```python
from build123d import *

# Parameters (mm, degrees)
SKETCH_3_R      = 1.6
EXTRUDE_2_DEPTH = 4


with BuildPart() as part:
    # Эскиз3 → Бобышка-Вытянуть2 (new body)
    # profile 1 of 6: a face of its own
    with BuildSketch(Plane.XY):
        Polygon((-16, -10), (-70, -10), (-70, -15.5), (-57.5, -15.5), (-57.5, -36.5), (-70, -36.5), (-70, -42), (-16, -42), (-16, -36.5), (-28.5, -36.5), (-28.5, -15.5), (-16, -15.5), align=None)
        with Locations((-66, -39)):
            Circle(SKETCH_3_R, mode=Mode.SUBTRACT)
        with Locations((-54, -26)):
            Circle(SKETCH_3_R, mode=Mode.SUBTRACT)
        with Locations((-20, -39)):
            Circle(SKETCH_3_R, mode=Mode.SUBTRACT)
        with Locations((-32, -26)):
            Circle(SKETCH_3_R, mode=Mode.SUBTRACT)
        with Locations((-66, -13)):
            Circle(SKETCH_3_R, mode=Mode.SUBTRACT)
        with Locations((-20, -13)):
            Circle(SKETCH_3_R, mode=Mode.SUBTRACT)
    # profile 2 of 6: a face of its own
    with BuildSketch(Plane.XY):
        Polygon((70, -10), (43, -10), (43, -42), (70, -42), (70, -36.5), (57.5, -36.5), (57.5, -15.5), (70, -15.5), align=None)
        with Locations((66, -39)):
            Circle(SKETCH_3_R, mode=Mode.SUBTRACT)
        with Locations((54, -26)):
            Circle(SKETCH_3_R, mode=Mode.SUBTRACT)
        with Locations((66, -13)):
            Circle(SKETCH_3_R, mode=Mode.SUBTRACT)
    # profile 3 of 6: a face of its own
    with BuildSketch(Plane.XY):
        Polygon((-70, 10), (-70, -10), (-16, -10), (43, -10), (70, -10), (70, 10), (43, 10), (-16, 10), (-43, 10), align=None)
    # profile 4 of 6: a face of its own
    with BuildSketch(Plane.XY):
        Polygon((-43, 42), (-43, 10), (-16, 10), (-16, 15.5), (-28.5, 15.5), (-28.5, 36.5), (-16, 36.5), (-16, 42), align=None)
        with Locations((-20, 13)):
            Circle(SKETCH_3_R, mode=Mode.SUBTRACT)
        with Locations((-32, 26)):
            Circle(SKETCH_3_R, mode=Mode.SUBTRACT)
        with Locations((-20, 39)):
            Circle(SKETCH_3_R, mode=Mode.SUBTRACT)
    # profile 5 of 6: a face of its own
    with BuildSketch(Plane.XY):
        Polygon((-70, 15.5), (-70, 10), (-43, 10), (-43, 42), (-70, 42), (-70, 36.5), (-57.5, 36.5), (-57.5, 15.5), align=None)
        with Locations((-66, 13)):
            Circle(SKETCH_3_R, mode=Mode.SUBTRACT)
        with Locations((-54, 26)):
            Circle(SKETCH_3_R, mode=Mode.SUBTRACT)
        with Locations((-66, 39)):
            Circle(SKETCH_3_R, mode=Mode.SUBTRACT)
    # profile 6 of 6: a face of its own
    with BuildSketch(Plane.XY):
        Polygon((43, 10), (70, 10), (70, 15.5), (57.5, 15.5), (57.5, 36.5), (70, 36.5), (70, 42), (43, 42), align=None)
        with Locations((66, 13)):
            Circle(SKETCH_3_R, mode=Mode.SUBTRACT)
        with Locations((54, 26)):
            Circle(SKETCH_3_R, mode=Mode.SUBTRACT)
        with Locations((66, 39)):
            Circle(SKETCH_3_R, mode=Mode.SUBTRACT)
    extrude(amount=EXTRUDE_2_DEPTH)


solid = part.part
```
Model file for the job. Use its own axes, mm. A direction names the side the tool comes from. Coordinates: 2 decimals unless noted, no trailing zeros. Write each loop counter-clockwise with the first axis right and the second up, starting at its lowest first coordinate (ties: lowest second). Pieces come first, ordered by that corner, then holes. Notation, with made-up numbers: (-35.75, 77) - (-19.75, 77) arc R9 cw to (-19.75, 81) - close; hole circle Ø2 at (-7.5, 12). An arc over 180 degrees is marked (long way). One line per item, written item: value. Start each with the question number.
1. Mould opens along Y. For faces 1 (the flat face through (-43, -42, 2)), 2 (the cylindrical face through (-64.52, 38.39, 1.97)), 3 (the flat face through (-16, -39, 2)) say: released by +Y, released by -Y, zero draft, split by the parting line, or undercut.
2. Slice it at A-A (x = 54). Write the cut outline in (y, z).
3. Tool access for faces 4 (the flat face through (-28.5, -26, 2)), 5 (the flat face through (70, 0, 2)), 6 (the flat face through (57, 42, 2)), 7 (the flat face through (43, 26, 2)), 8 (the flat face through (-16, -13, 2)): list every direction of +Z, -Z, +X, -X, +Y, -Y with a clear straight run to the whole face (end or side of a thin tool).
4. Slice it at B-B (y = 26). Write the cut outline in (x, z).
5. Probe line 1 (Y direction, x = -54, z = 1.35); line 2 (X direction, y = -10.5, z = 1.1); line 3 (X direction, y = -12, z = 0.65). List the from-to ranges inside material, lowest first. Write a range as from..to.
6. Flat gauge pin, fed straight in: pin 1 (1.2 mm diameter, centred on x = -0.5, z = 3, fed in from +Y). Where does the tip first touch, or does it go through?
7. Slice it at D-D (z = 3.1). Count the separate pieces of the cut face and the enclosed holes in it, plus the area to 3 significant figures.
8. Slice it at C-C (y = -39). Write the cut outline in (x, z), plus the area to 3 significant figures.
Answers below:
1. face 1: released by -Y
1. face 2: undercut
1. face 3: zero draft
2. outline: (-42, 0) - (-27.6, 0) - (-27.6, 4) - (-42, 4) - close; (-24.4, 0) - (24.4, 0) - (24.4, 4) - (-24.4, 4) - close; (27.6, 0) - (42, 0) - (42, 4) - (27.6, 4) - close
3. face 4: +Z, -Z
3. face 5: +Z, -Z, +X, +Y, -Y
3. face 6: +Z, -Z, +X, -X, +Y
3. face 7: +Z, -Z, +Y
3. face 8: +Z, -Z, -Y
4. outline: (-57.5, 0) - (-55.6, 0) - (-55.6, 4) - (-57.5, 4) - close; (-52.4, 0) - (-33.6, 0) - (-33.6, 4) - (-52.4, 4) - close; (-30.4, 0) - (-28.5, 0) - (-28.5, 4) - (-30.4, 4) - close; (43, 0) - (52.4, 0) - (52.4, 4) - (43, 4) - close; (55.6, 0) - (57.5, 0) - (57.5, 4) - (55.6, 4) - close
5. line 1: y = -42..-27.6, -24.4..24.4, 27.6..42
5. line 2: x = -70..-16, 43..70
5. line 3: x = -70..-67.25, -64.75..-21.25, -18.75..-16, 43..64.75, 67.25..70
6. pin 1: stops at y = 10
7. separate pieces: 1
7. enclosed holes: 18
7. area: 6,260 mm^2
8. outline: (-70, 0) - (-67.6, 0) - (-67.6, 4) - (-70, 4) - close; (-64.4, 0) - (-21.6, 0) - (-21.6, 4) - (-64.4, 4) - close; (-18.4, 0) - (-16, 0) - (-16, 4) - (-18.4, 4) - close; (43, 0) - (64.4, 0) - (64.4, 4) - (43, 4) - close; (67.6, 0) - (70, 0) - (70, 4) - (67.6, 4) - close
8. area: 286 mm^2
